For this review, take the finished solid that the model builds, in its own axes (mm). Round coordinates to 2 decimals unless told otherwise and drop trailing zeros. Write each loop counter-clockwise with the first axis right and the second up, starting at its lowest first coordinate (ties: lowest second). Pieces come first, ordered by that corner, then holes. Notation, with made-up numbers: M -8,20.25 L 48,20.25 A11 ccw 48,41.25 Z; hole C -11.5,-28.75 d10. An arc over 180 degrees is marked long. One line per question, with ' | ' between items.
```python
from build123d import *

# Parameters (mm, degrees)
SKETCH1_R           = 1.7
BOSS_EXTRUDE1_DEPTH = 177.8
CHAMFER1_SIZE       = 0.5


with BuildPart() as part:
    # Sketch1 → Boss-Extrude1 (new body)
    with BuildSketch(Plane.XY):
        with BuildLine():
            Line((-0.97, 18.75), (0.97, 18.75))
            ThreePointArc((0.97, 18.75), (4.562102448, 17.262102448), (6.05, 13.67))
            Line((6.05, 13.67), (6.05, -18.75))
            Line((6.05, -18.75), (-6.05, -18.75))
            Line((-6.05, -18.75), (-6.05, 13.67))
            ThreePointArc((-6.05, 13.67), (-4.562102448, 17.262102448), (-0.97, 18.75))
        make_face()
        with Locations((0, 13)):
            Circle(SKETCH1_R, mode=Mode.SUBTRACT)
        with Locations((0, -7.32)):
            Circle(SKETCH1_R, mode=Mode.SUBTRACT)
    extrude(amount=BOSS_EXTRUDE1_DEPTH)

    # Chamfer1
    chamfer1_edges = [part.edges().sort_by_distance(p)[0] for p in [
        (6.05, -18.75, 88.9),
        (-6.05, -18.75, 88.9),
        (0, 18.75, 177.8),
        (-4.562102448, 17.262102448, 177.8),
        (-6.05, -2.54, 177.8),
        (6.05, -2.54, 177.8),
        (-6.05, -2.54, 0),
        (-4.562102448, 17.262102448, 0),
        (0, 18.75, 0),
        (4.562102448, 17.262102448, 0),
        (6.05, -2.54, 0),
        (4.562102448, 17.262102448, 177.8),
    ]]
    chamfer(chamfer1_edges, length=CHAMFER1_SIZE)


solid = part.part
```
Item 1: To check wall thickness, follow line 1 along Y through (x, z) = (0, 101.5); line 2 along Y through (x, z) = (1, 159); line 3 along X through (y, z) = (-7, 110). State the ranges of each line that lie inside material, in increasing order. Write a range as from..to.
Results:
line 1: -18.75..-9.02, -5.62..11.3, 14.7..18.75 | line 2: -18.75..-8.69, -5.95..11.63, 14.37..18.75 | line 3: -6.05..-1.67, 1.67..6.05
Item 2: Mouldability with a two-part tool opening along X and no side actions: class faces 1 (the face through (-0.221, 14.686, 87.655)), 2 (the face through (-4.341, 16.967, 177.665)), 3 (the face through (4.267, 17.041, 0.135)) as +X half, -X half, draft (parallel to the pull), parting line (faces both ways), or undercut.
Results:
face 1: undercut | face 2: -X half | face 3: +X half
Item 3: Take a section at B-B (z = 83.5). Write out the cut boundary in (x, y), then the cut area to 3 significant figures.
Results:
outline: M -6.05,-18.25 L -5.55,-18.75 L 5.55,-18.75 L 6.05,-18.25 L 6.05,13.67 A5.08 ccw 0.97,18.75 L -0.97,18.75 A5.08 ccw -6.05,13.67 Z; hole C 0,-7.32 d3.4; hole C 0,13 d3.4 | area: 424 mm2
Item 4: Take a section at A-A (y = -7.32). Write out the cut boundary in (x, z).
Results:
outline: M -6.05,0.5 L -5.55,0 L -1.7,0 L -1.7,177.8 L -5.55,177.8 L -6.05,177.3 Z; M 1.7,0 L 5.55,0 L 6.05,0.5 L 6.05,177.3 L 5.55,177.8 L 1.7,177.8 Z
